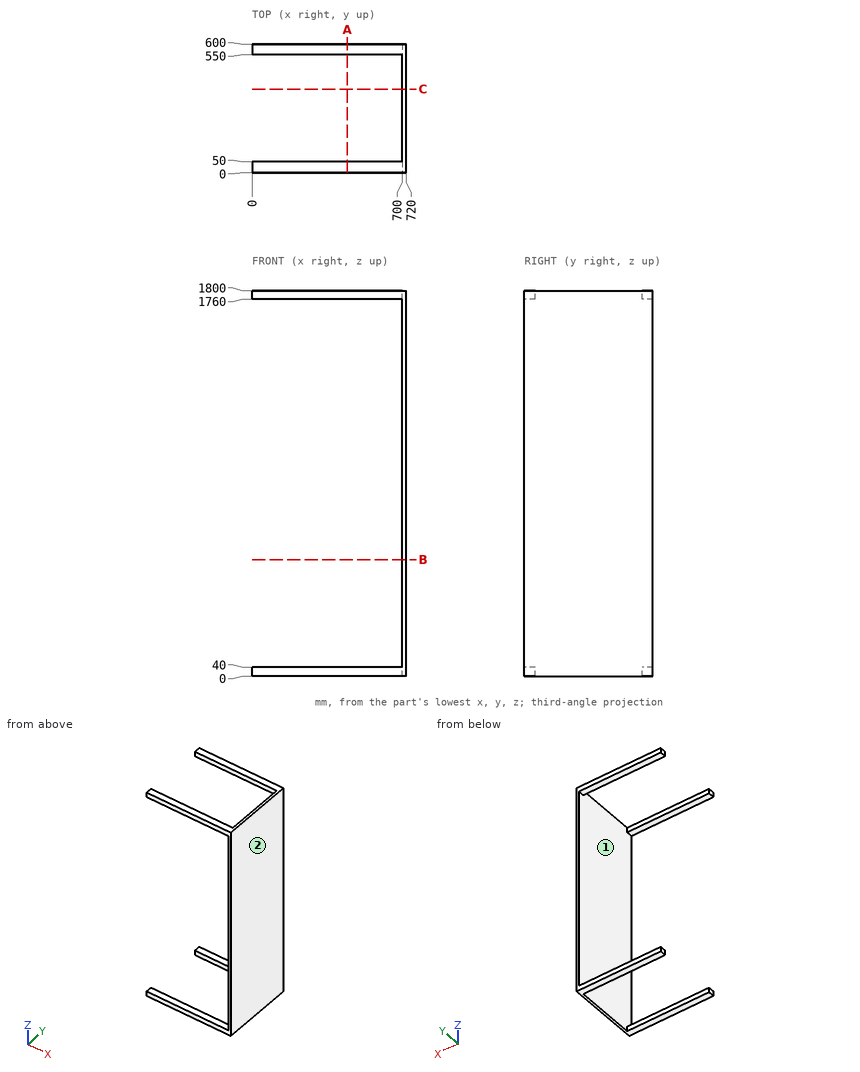
Answer from the drawing. Dimensions are ordinates in mm from the lowest x, y and z of the part. Round coordinates to 2 decimals unless told otherwise and drop trailing zeros. Loops run counter-clockwise (first coordinate to the right, second up) from the corner with the lowest first, then second, coordinate; pieces in that order, holes last.
(1) The part is cut by section C-C, the plane y = 389. Give the vertices of the cut face in (x, z), and give its area (3 significant figures).
Computed values:
outline: (700, 0) - (720, 0) - (720, 1800) - (700, 1800) - close
area: 36,000 mm2
(2) The part is cut by section B-B, the plane z = 543.5. Give the vertices of the cut face in (x, y), and give its area (3 significant figures).
Computed values:
outline: (700, 0) - (720, 0) - (720, 600) - (700, 600) - close
area: 12,000 mm2
(3) Find the intervals of material crossed by L1, parallel to Z at x = 285.5, y = 553; L2, parallel to X at y = 203, z = 569, in increasing order.
Computed values:
L1: z = 0 to 40, 1760 to 1800
L2: x = 700 to 720
(4) Each of these flat-tipped pins is pushed along its axis until it touches: P1, Ø2, axis at y = 285.5, z = 745.5, coming from the -X side; P2, Ø20, axis at x = 248.5, z = 28, coming from the -Y side. Where does it stop, or does it pass through?
Computed values:
P1: stops at x = 700
P2: stops at y = 0
(5) The part is cut by section A-A, the plane x = 445. Give the vertices of the cut face in (y, z), and give its area (3 significant figures).
Computed values:
outline: (0, 0) - (50, 0) - (50, 40) - (0, 40) - close; (0, 1760) - (50, 1760) - (50, 1800) - (0, 1800) - close; (550, 0) - (600, 0) - (600, 40) - (550, 40) - close; (550, 1760) - (600, 1760) - (600, 1800) - (550, 1800) - close
area: 8,000 mm2
(6) The mould has two halves that part along Z. Classify the marked faces 1 and 2: pulls with the +Z half, pulls with the -Z half, needs draft (parallel to the pull), parting line crosses it, or undercut.
Computed values:
face 1: undercut
face 2: needs draft
